from build123d import *

# Parameters (mm, degrees)
F0_R     = 20.5
F1_DEPTH = 3
F2_W     = 10
F2_H     = 3
F2_W_2   = 3
F2_H_2   = 10
F3_DEPTH = 3


with BuildPart() as f1:
    # F0 (on Top) → F1 (new body)
    with BuildSketch(Plane.XY):
        Polygon((-85.136861, 107.09559), (-107.005506, 107.09559), (-107.005506, -106.90441), (106.994494, -106.90441), (106.994494, 107.09559), align=None)
        with Locations((-0.005506, 0.09559)):
            Circle(F0_R, mode=Mode.SUBTRACT)
    extrude(amount=F1_DEPTH)

    # F2 (on face) → F3 (join)
    with BuildSketch(Plane.XY.offset(3)):
        with Locations((-5.005506, 108.59559)):
            Rectangle(F2_W, F2_H)
        with Locations((4.994494, 108.59559)):
            Rectangle(F2_W, F2_H)
        with Locations((-95.005506, 108.59559)):
            Rectangle(F2_W, F2_H)
        with Locations((94.994494, 108.59559)):
            Rectangle(F2_W, F2_H)
        with Locations((4.994494, -108.40441)):
            Rectangle(F2_W, F2_H)
        with Locations((-5.005506, -108.40441)):
            Rectangle(F2_W, F2_H)
        with Locations((-95.005506, -108.40441)):
            Rectangle(F2_W, F2_H)
        with Locations((94.994494, -108.40441)):
            Rectangle(F2_W, F2_H)
        with Locations((-108.505506, -4.90441)):
            Rectangle(F2_W_2, F2_H_2)
        with Locations((-108.505506, 5.09559)):
            Rectangle(F2_W_2, F2_H_2)
        with Locations((-108.505506, -94.90441)):
            Rectangle(F2_W_2, F2_H_2)
        with Locations((-108.505506, 95.09559)):
            Rectangle(F2_W_2, F2_H_2)
        with Locations((108.494494, 5.09559)):
            Rectangle(F2_W_2, F2_H_2)
        with Locations((108.494494, -4.90441)):
            Rectangle(F2_W_2, F2_H_2)
        with Locations((108.494494, 95.09559)):
            Rectangle(F2_W_2, F2_H_2)
        with Locations((108.494494, -94.90441)):
            Rectangle(F2_W_2, F2_H_2)
    extrude(amount=-F3_DEPTH)


solid = f1.part
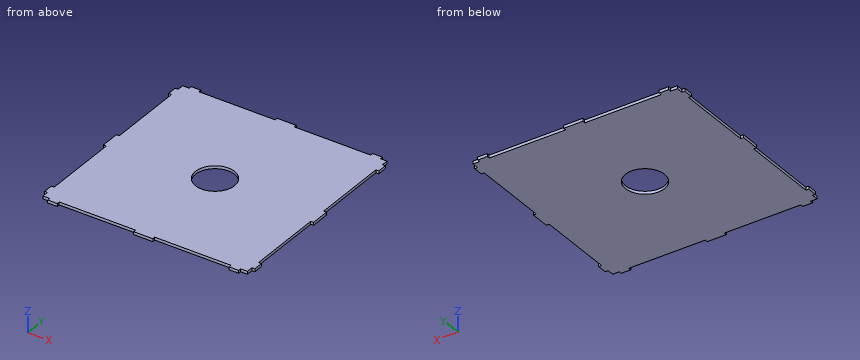
Here's how the part is built. I have some questions about the finished solid (model axes, mm). Round coordinates to 2 decimals unless told otherwise and drop trailing zeros. Order: outer loops, then holes, each group sorted by start corner. A loop starts at its lowest first (then second) coordinate and runs counter-clockwise, first axis right, second up. Notation, with made-up numbers: (-16.75, 68.25) -> (-1.75, 68.25) arc R10 ccw to (-1.75, 78.25) -> close; hole circle Ø11 at (84, 66). An arc over 180 degrees is marked (long way). Return JSON: item names as keys, results as strings.
Q1. If we section it at A-A on x = -6.5: List the corners of the cut face in (y, z) for me, plus the area to 3 significant figures.
Filled sheet:
{"outline": "(-109.9, 0) -> (-19.35, 0) -> (-19.35, 3) -> (-109.9, 3) -> close; (19.54, 0) -> (110.1, 0) -> (110.1, 3) -> (19.54, 3) -> close", "area": "543 mm^2"}
Q2. If we section it at C-C on x = -59.5: List the corners of the cut face in (y, z) for me, plus the area to 3 significant figures.
Filled sheet:
{"outline": "(-106.9, 0) -> (107.1, 0) -> (107.1, 3) -> (-106.9, 3) -> close", "area": "642 mm^2"}
Q3. I need wall thicknesses on line 1 along X through (y, z) = (-67, 1); line 2 along Y through (x, z) = (71, 0.85); line 3 along X through (y, z) = (-4, 1.8). Which ranges of each line are inside material? Lowest first, please. Write a range as from..to.
Filled sheet:
{"line 1": "x = -107.01..106.99", "line 2": "y = -106.9..107.1", "line 3": "x = -110.01..-20.09, 20.08..109.99"}
Q4. For pin 1 Ø1.5 at (y, z) = (-108, 1.5) entering from -X; pin 2 Ø0.9 at (y, z) = (-53, 1) entering from +X; pin 3 Ø0.9 at (y, z) = (108, 2) entering from +X, each with a flat end and sliding along its axis, tell me the tip position at first contact or that it passes through.
Filled sheet:
{"pin 1": "stops at x = -100.01", "pin 2": "stops at x = 106.99", "pin 3": "stops at x = 99.99"}
Q5. If we section it at B-B on y = 74.5: List the corners of the cut face in (x, z) for me, plus the area to 3 significant figures.
Filled sheet:
{"outline": "(-107.01, 0) -> (106.99, 0) -> (106.99, 3) -> (-107.01, 3) -> close", "area": "642 mm^2"}
